Design review of the part built by this model. Coordinates are the model's own, in mm. Face numbers are marked on the shaded views. Coordinates: 2 decimals unless noted, no trailing zeros. Loops run counter-clockwise (first coordinate to the right, second up) from the corner with the lowest first, then second, coordinate; pieces in that order, holes last.
Q1. Add section D-D on x = 36.5. Give the boundary of the cut face in (y, z).
Q2. Draft analysis for pull direction X (two halves, no side actions). For the marked faces 1, 2, 3 and 4, state which applies: released by +X, released by -X, zero draft, split by the parting line, or undercut.
Q3. For P1, Ø9, axis at x = -30, z = 0, coming from the +Y side; P2, Ø1, axis at y = 3, z = -6.5, coming from the +X side; P3, Ø3, axis at y = 0.5, z = -6.5, coming from the +X side, all flat-tipped, find the tip position at first contact; note any pin that passes through.
Q4. Add section B-B on x = 27.5. Give the boundary of the cut face in (y, z).
Q5. Wall thickness on probe 1 along X at (y, z) = (-1.5, 0); probe 2 along X at (y, z) = (3.5, -4.5); probe 3 along Z at (x, y) = (-33.5, 3): over which ranges is each line inside the solid? List them lowest first.
Q6. Add section C-C on y = 1.25. Give the boundary of the cut face in (x, z).
Q7. Add section A-A on z = 0. Give the boundary of the cut face in (x, y), and give its area (3 significant figures).
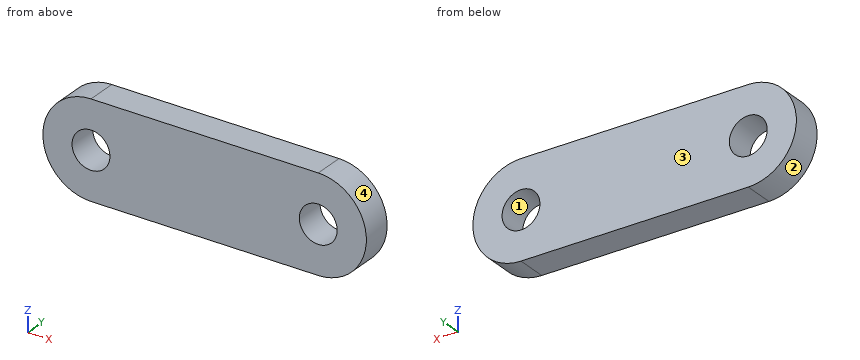
```python
from build123d import *

# Parameters (mm, degrees)
ESBO_O1_R                = 5
RESSALTO_EXTRUS_O1_DEPTH = 4


with BuildPart() as part:
    # Esboço1 → Ressalto-extrusão1 (new, symmetric)
    with BuildSketch(Plane(origin=(0, 0, 0), x_dir=(1, 0, 0), z_dir=(0, 1, 0))):
        with BuildLine():
            Line((-30, 12.7), (30, 12.7))
            ThreePointArc((30, 12.7), (42.7, 0), (30, -12.7))
            Line((30, -12.7), (-30, -12.7))
            ThreePointArc((-30, -12.7), (-42.7, 0), (-30, 12.7))
        make_face()
        with Locations(Location((30, 0, 0), (0, 0, 270))):
            Circle(ESBO_O1_R, mode=Mode.SUBTRACT)
        with Locations(Location((-30, 0, 0), (0, 0, 270))):
            Circle(ESBO_O1_R, mode=Mode.SUBTRACT)
    extrude(amount=RESSALTO_EXTRUS_O1_DEPTH, both=True)


solid = part.part
```
Entries:
1. outline: (-4, -10.91) - (4, -10.91) - (4, 10.91) - (-4, 10.91) - close
2. face 1: undercut
2. face 2: released by -X
2. face 3: zero draft
2. face 4: released by +X
3. P1: passes through
3. P2: stops at x = 41.19
3. P3: stops at x = 41.67
4. outline: (-4, -12.7) - (4, -12.7) - (4, -4.33) - (-4, -4.33) - close; (-4, 4.33) - (4, 4.33) - (4, 12.7) - (-4, 12.7) - close
5. probe 1: x = -42.7 to -35, -25 to 25, 35 to 42.7
5. probe 2: x = -41.88 to -32.18, -27.82 to 27.82, 32.18 to 41.88
5. probe 3: z = -12.21 to -3.57, 3.57 to 12.21
6. outline: (-30, -12.7) - (30, -12.7) arc R12.7 ccw to (30, 12.7) - (-30, 12.7) arc R12.7 ccw to start; hole circle Ø10 at (-30, 0); hole circle Ø10 at (30, 0)
7. outline: (-42.7, -4) - (-35, -4) - (-35, 4) - (-42.7, 4) - close; (-25, -4) - (25, -4) - (25, 4) - (-25, 4) - close; (35, -4) - (42.7, -4) - (42.7, 4) - (35, 4) - close
7. area: 523 mm2
